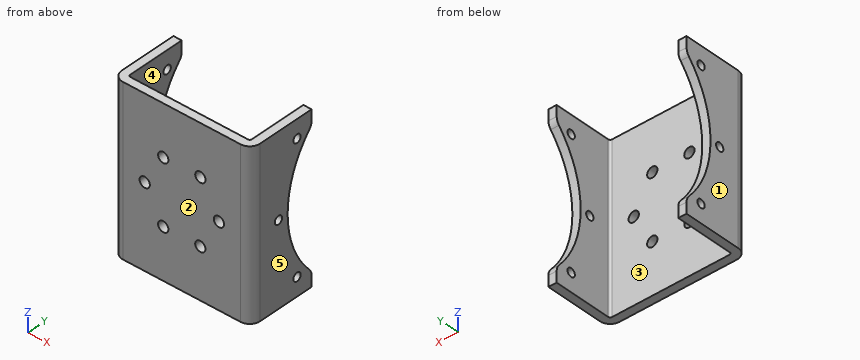
from build123d import *

# Parameters (mm, degrees)
SM_BASE_FLANGE_1_DEPTH   = 80
CUT_EXTRUDE_3_DEPTH      = 109.305124532
CUT_EXTRUDE_3_DEPTH_BACK = 109.305124532
SKETCH_6_R               = 48
SKETCH_6_R_2             = 2
FILLET_1_R               = 5
SKETCH_9_R               = 2.5
CUT_EXTRUDE_4_DEPTH      = 93.796821066


# Sheet-metal steps are written as plain solids
with BuildPart() as part:
    # Sketch 1 → Базовая кромка1 (new body)
    with BuildSketch(Plane.XY):
        with BuildLine():
            Line((-29.5, 29), (-29.5, 1))
            ThreePointArc((-29.5, 1), (-29.207106781, 0.292893219), (-28.5, 0))
            Line((-28.5, 0), (28.5, 0))
            ThreePointArc((28.5, 0), (29.207106781, 0.292893219), (29.5, 1))
            Line((29.5, 1), (29.5, 29))
            Line((29.5, 29), (33.5, 29))
            Line((33.5, 29), (33.5, 1))
            ThreePointArc((33.5, 1), (32.035533906, -2.535533906), (28.5, -4))
            Line((28.5, -4), (-28.5, -4))
            ThreePointArc((-28.5, -4), (-32.035533906, -2.535533906), (-33.5, 1))
            Line((-33.5, 1), (-33.5, 29))
            Line((-33.5, 29), (-29.5, 29))
        make_face()
    extrude(amount=SM_BASE_FLANGE_1_DEPTH)

    # Эскиз6 → Вырез-Вытянуть3 (cut, two sides: drawn at the far end of the back side and taken through both)
    with BuildSketch(Plane.ZY.offset(33.5).offset(-CUT_EXTRUDE_3_DEPTH_BACK)):
        with Locations((40, 64)):
            Circle(SKETCH_6_R)
        with Locations((40, 11)):
            Circle(SKETCH_6_R_2)
        with Locations((8.847381628, 21.122099298)):
            Circle(SKETCH_6_R_2)
        with Locations((71.152618372, 21.122099298)):
            Circle(SKETCH_6_R_2)
    extrude(amount=CUT_EXTRUDE_3_DEPTH + CUT_EXTRUDE_3_DEPTH_BACK, mode=Mode.SUBTRACT)

    # Скругление1
    fillet_1_edges = [part.edges().sort_by_distance(p)[0] for p in [
        (31.5, 29, 7.151864589),
        (31.5, 29, 72.848135411),
        (-31.5, 29, 7.151864589),
        (-31.5, 29, 72.848135411),
    ]]
    fillet(fillet_1_edges, radius=FILLET_1_R)

    # Эскиз9 → Вырез-Вытянуть4 (cut, through all)
    with BuildSketch(Plane.XZ.offset(4)):
        with Locations((18, 40)):
            Circle(SKETCH_9_R)
        with Locations((9, 24.411542732)):
            Circle(SKETCH_9_R)
        with Locations((-9, 24.411542732)):
            Circle(SKETCH_9_R)
        with Locations((-18, 40)):
            Circle(SKETCH_9_R)
        with Locations((-9, 55.588457268)):
            Circle(SKETCH_9_R)
        with Locations((9, 55.588457268)):
            Circle(SKETCH_9_R)
    extrude(amount=-CUT_EXTRUDE_4_DEPTH, mode=Mode.SUBTRACT)


solid = part.part
Check sheet for the modelled part. Datum: model origin and axes. Units: mm. Face numbers are marked on the shaded views. A direction names the side the tool comes from. Coordinates: 2 decimals unless noted, no trailing zeros. Write each loop counter-clockwise with the first axis right and the second up, starting at its lowest first coordinate (ties: lowest second). Pieces come first, ordered by that corner, then holes. Notation, with made-up numbers: M 89.25,22 L 112.25,22 A30 cw 112.25,47 Z; hole C -33,67 d6. An arc over 180 degrees is marked long. Answer as CSV lines item,"result".
Q1. Set-up check for the marked faces 4 and 5: record each of +Z, -Z, +X, -X, +Y, -Y from which the full face is reachable in a straight line by a thin tool's end or side.
Check result:
face 4,"+Z, -Z, +Y"
face 5,"+Z, -Z, +X, +Y, -Y"
Q2. Go/stop test with flat-tipped pins: pin 1 (8 mm diameter, centred on x = 25, y = 21, fed in from +Z); pin 2 (1.5 mm diameter, centred on x = 0.5, z = 55, fed in from +Y). Record where each tip stops, or that it passes through.
Check result:
pin 1,"through"
pin 2,"y = 0"
Q3. Cross-section at C-C (x = -9). Record the boundary of the cut face in (y, z).
Check result:
outline,"M -4,0 L 0,0 L 0,21.91 L -4,21.91 Z; M -4,26.91 L 0,26.91 L 0,53.09 L -4,53.09 Z; M -4,58.09 L 0,58.09 L 0,80 L -4,80 Z"
Q4. Cross-section at A-A (y = 15). Record the boundary of the cut face in (x, z), then the cut area to 3 significant figures.
Check result:
outline,"M -33.5,0 L -29.5,0 L -29.5,80 L -33.5,80 Z; M 29.5,0 L 33.5,0 L 33.5,80 L 29.5,80 Z"
area,"640 mm^2"
Q5. Mould release check, pull along X, two halves, no side actions. Record for the marked faces 1, 2 and 3: released by +X, released by -X, zero draft, split by the parting line, or undercut.
Check result:
face 1,"released by -X"
face 2,"zero draft"
face 3,"undercut"
Q6. Cross-section at B-B (z = 40). Record the boundary of the cut face in (x, y), then the cut area to 3 significant figures.
Check result:
outline,"M -33.5,1 A5 ccw -28.5,-4 L -20.5,-4 L -20.5,0 L -28.5,0 A1 cw -29.5,1 L -29.5,9 L -33.5,9 Z; M -33.5,13 L -29.5,13 L -29.5,16 L -33.5,16 Z; M -15.5,-4 L 15.5,-4 L 15.5,0 L -15.5,0 Z; M 20.5,-4 L 28.5,-4 A5 ccw 33.5,1 L 33.5,9 L 29.5,9 L 29.5,1 A1 cw 28.5,0 L 20.5,0 Z; M 29.5,13 L 33.5,13 L 33.5,16 L 29.5,16 Z"
area,"314 mm^2"
Q7. Cross-section at D-D (x = 18). Record the boundary of the cut face in (y, z).
Check result:
outline,"M -4,0 L 0,0 L 0,37.5 L -4,37.5 Z; M -4,42.5 L 0,42.5 L 0,80 L -4,80 Z"
Q8. Material ranges on probe 1 along X at (y, z) = (3.5, 52); probe 2 along Y at (x, z) = (22, 26); probe 3 along Z at (x, y) = (32, 11), recorded low to high. Write a range as from..to.
Check result:
probe 1,"-33.5..-29.5, 29.5..33.5"
probe 2,"-4..0"
probe 3,"0..38, 42..80"
